The model under review builds one solid part; all positions refer to its coordinate system, in mm. A direction names the side the tool comes from. Round coordinates to 2 decimals unless told otherwise and drop trailing zeros. Order: outer loops, then holes, each group sorted by start corner. A loop starts at its lowest first (then second) coordinate and runs counter-clockwise, first axis right, second up. Notation, with made-up numbers: (-10.5, 33.25) -> (2.5, 33.25) arc R27 cw to (2.5, 61.25) -> close; hole circle Ø8 at (21, -24). An arc over 180 degrees is marked (long way). Use a Markdown table: item, result. Add a question column.
```python
from build123d import *

# Parameters (mm, degrees)
F1_DEPTH = 6.35


with BuildPart() as f1:
    # F0 (on Top) → F1 (new body)
    with BuildSketch(Plane.XY):
        Polygon((57.15, 132.08), (57.15, 146.05), (24.13, 146.05), (24.13, 152.4), (3.81, 152.4), (3.81, 146.05), (-16.51, 146.05), (-16.51, 152.4), (-36.83, 152.4), (-36.83, 146.05), (-57.15, 146.05), (-57.15, 132.08), (-63.5, 132.08), (-63.5, 111.76), (-57.15, 111.76), (-57.15, 91.44), (-63.5, 91.44), (-63.5, 71.12), (-57.15, 71.12), (-57.15, 50.8), (-63.5, 50.8), (-63.5, 30.48), (-57.15, 30.48), (-57.15, 10.16), (-63.5, 10.16), (-63.5, -10.16), (-57.15, -10.16), (-57.15, -30.48), (-63.5, -30.48), (-63.5, -50.8), (-57.15, -50.8), (-57.15, -71.12), (-63.5, -71.12), (-63.5, -91.44), (-57.15, -91.44), (-57.15, -111.76), (-63.5, -111.76), (-63.5, -132.08), (-57.15, -132.08), (-57.15, -146.05), (-36.83, -146.05), (-36.83, -152.4), (-16.51, -152.4), (-16.51, -146.05), (3.81, -146.05), (3.81, -152.4), (24.13, -152.4), (24.13, -146.05), (57.15, -146.05), (57.15, -132.08), (63.5, -132.08), (63.5, -111.76), (57.15, -111.76), (57.15, -91.44), (63.5, -91.44), (63.5, -71.12), (57.15, -71.12), (57.15, -50.8), (63.5, -50.8), (63.5, -30.48), (57.15, -30.48), (57.15, -10.16), (63.5, -10.16), (63.5, 10.16), (57.15, 10.16), (57.15, 30.48), (63.5, 30.48), (63.5, 50.8), (57.15, 50.8), (57.15, 71.12), (63.5, 71.12), (63.5, 91.44), (57.15, 91.44), (57.15, 111.76), (63.5, 111.76), (63.5, 132.08), align=None)
    extrude(amount=F1_DEPTH)


solid = f1.part
```
Q1. Add section A-A, the plane y = 108.5. Give the boundary of the cut face in (x, z).
Q2. For pin 1 (1.5 mm diameter, centred on x = 16.5, y = -111, fed in from -Z); pin 2 (1 mm diameter, centred on y = -69, z = 4.5, fed in from +X); pin 3 (3 mm diameter, centred on y = -150, z = 2, fed in from -X); pin 4 (1.9 mm diameter, centred on x = -59, z = 3.5, fed in from -Y), all flat-tipped, find the tip position at first contact; note any pin that passes through.
Q3. For faces 4 (the face through (-63.5, -40, 3)), 5 (the face through (41, 146.05, 3)), 6 (the face through (60, -71.12, 3)), 7 (the face through (-36.83, 149, 3)), 8 (the face through (-60, 91.44, 3)), list the 3-axis set-ups (+Z, -Z, +X, -X, +Y, -Y) from which the entire face can be reached by the end or side of a thin tool; tool diameter is ignored.
Q4. Add section B-B, the plane x = -5. Give the boundary of the cut face in (y, z), then the cut area to 3 significant figures.
Q5. Draft analysis for pull direction Y (two halves, no side actions). For faces 1 (the face through (-60, -91.44, 3)), 2 (the face through (-57.15, -139, 3)), 3 (the face through (-27, 152.4, 3)), state which applies: released by +Y, released by -Y, zero draft, split by the parting line, or undercut.
Q6. To check wall thickness, follow line 1 along X through (y, z) = (17, 2.25); line 2 along Y through (x, z) = (47.5, 2). State the ranges of each line that lie inside material, in increasing order.
Return value:
| question | item | result |
|---|---|---|
| 1 | outline | (-57.15, 0) -> (57.15, 0) -> (57.15, 6.35) -> (-57.15, 6.35) -> close |
| 2 | pin 1 | z = 0 |
| 2 | pin 2 | x = 57.15 |
| 2 | pin 3 | x = -36.83 |
| 2 | pin 4 | y = -132.08 |
| 3 | face 4 | +Z, -Z, -X, +Y, -Y |
| 3 | face 5 | +Z, -Z, +X, +Y |
| 3 | face 6 | +Z, -Z, +X |
| 3 | face 7 | +Z, -Z, -X, +Y |
| 3 | face 8 | +Z, -Z, -X |
| 4 | outline | (-146.05, 0) -> (146.05, 0) -> (146.05, 6.35) -> (-146.05, 6.35) -> close |
| 4 | area | 1,850 mm² |
| 5 | face 1 | undercut |
| 5 | face 2 | zero draft |
| 5 | face 3 | released by +Y |
| 6 | line 1 | -57.15 to 57.15 |
| 6 | line 2 | -146.05 to 146.05 |
